from build123d import *

# Parameters (mm, degrees)
SKETCH1_R           = 32.5
BOSS_EXTRUDE1_DEPTH = 10
BOSS_EXTRUDE2_DEPTH = 5.4
SKETCH3_R           = 7
CUT_EXTRUDE1_DEPTH  = 49.473291615


with BuildPart() as part:
    # Sketch1 → Boss-Extrude1 (new body)
    with BuildSketch(Plane(origin=(0, 0, 0), x_dir=(1, 0, 0), z_dir=(0, 1, 0))):
        with Locations(Location((0, 0, 0), (0, 0, 270))):
            Circle(SKETCH1_R)
    extrude(amount=BOSS_EXTRUDE1_DEPTH)

    # Sketch2 → Boss-Extrude2 (add)
    with BuildSketch(Plane(origin=(0, 10, 0), x_dir=(1, 0, 0), z_dir=(0, 1, 0))):
        with BuildLine():
            Line((2.725, 11.891777622), (2.725, 17.25))
            Line((2.725, 17.25), (-2.725, 17.25))
            Line((-2.725, 17.25), (-2.725, 11.891777622))
            ThreePointArc((-2.725, 11.891777622), (-8.62670273, 8.62670273), (-11.891777622, 2.725))
            Line((-11.891777622, 2.725), (-17.25, 2.725))
            Line((-17.25, 2.725), (-17.25, -2.725))
            Line((-17.25, -2.725), (-11.891777622, -2.725))
            ThreePointArc((-11.891777622, -2.725), (-8.62670273, -8.62670273), (-2.725, -11.891777622))
            Line((-2.725, -11.891777622), (-2.725, -17.25))
            Line((-2.725, -17.25), (2.725, -17.25))
            Line((2.725, -17.25), (2.725, -11.891777622))
            ThreePointArc((2.725, -11.891777622), (8.62670273, -8.62670273), (11.891777622, -2.725))
            Line((11.891777622, -2.725), (17.25, -2.725))
            Line((17.25, -2.725), (17.25, 2.725))
            Line((17.25, 2.725), (11.891777622, 2.725))
            ThreePointArc((11.891777622, 2.725), (8.62670273, 8.62670273), (2.725, 11.891777622))
        make_face()
    extrude(amount=BOSS_EXTRUDE2_DEPTH)

    # Sketch3 → Cut-Extrude1 (cut, through all)
    with BuildSketch(Plane(origin=(0, 15.4, 0), x_dir=(1, 0, 0), z_dir=(0, 1, 0))):
        with Locations(Location((0, 0, 0), (0, 0, 270))):
            Circle(SKETCH3_R)
    extrude(amount=-CUT_EXTRUDE1_DEPTH, mode=Mode.SUBTRACT)


solid = part.part
Part model, mm, in its own coordinate system. A direction names the side the tool comes from. Give positions to 0.01 mm unless a question says otherwise; leave off trailing zeros. Loops run counter-clockwise (first coordinate to the right, second up) from the corner with the lowest first, then second, coordinate; pieces in that order, holes last. Notation, with made-up numbers: M 88.5,-10 L 114.5,-10 A35 cw 114.5,22 Z; hole C 68.5,3 d3. An arc over 180 degrees is marked long. Put each result on its own line as item: value. Start each with the question number.
1) Saw through at C-C (y = 12). List the corners of the cut face in (x, z) (3 decimals), then the cut area to 3 significant figures.
2) Saw through at D-D (x = 16). List the corners of the cut face in (y, z) (3 decimals).
3) Flat gauge pins, fed straight in: pin 1 (4 mm diameter, centred on x = 25, z = 7.5, fed in from -Y); pin 2 (4.5 mm diameter, centred on y = 14, z = 14.5, fed in from -X) (3 decimals); pin 3 (2.5 mm diameter, centred on x = -14.5, y = 13.5, fed in from +Z) (3 decimals); pin 4 (3 mm diameter, centred on x = 3.5, y = 12, fed in from +Z). Where does each tip first touch, or does it go through?
4) Probe probe 1 along X at (y, z) = (7.75, 0); probe 2 along Y at (x, z) = (-1, -22.5); probe 3 along Z at (x, y) = (-3, 2.25). List the from-to ranges inside material, lowest first.
5) Pull direction Z, two halves, no side cores. Call faces 4 (the flat face through (-15, 13, 2.725)), 5 (the cylindrical face through (-6.834, 7.808, -1.517)), 6 (the flat face through (-15, 13, -2.725)), 7 (the flat face through (2.725, 13, 15)): +Z half, -Z half, draft (parallel to the pull), parting line (faces both ways), or undercut.
6) 3-axis set-ups, long thin cutter, end or side, ignore diameter. For faces 1 (the cylindrical face through (-8.694, 12.662, 8.559)), 2 (the flat face through (0, 13, 17.25)), 3 (the flat face through (17.25, 13, 0)): which of +Z, -Z, +X, -X, +Y, -Y reach the whole face in a straight line?
7) Saw through at A-A (z = 0). List the corners of the cut face in (x, y).
8) Saw through at B-B (x = 0). List the corners of the cut face in (y, z), then the cut area to 3 significant figures.
Numbers:
1. outline: M -17.25,-2.725 L -11.892,-2.725 A12.2 ccw -2.725,-11.892 L -2.725,-17.25 L 2.725,-17.25 L 2.725,-11.892 A12.2 ccw 11.892,-2.725 L 17.25,-2.725 L 17.25,2.725 L 11.892,2.725 A12.2 ccw 2.725,11.892 L 2.725,17.25 L -2.725,17.25 L -2.725,11.892 A12.2 ccw -11.892,2.725 L -17.25,2.725 Z; hole C 0,0 d14
1. area: 426 mm^2
2. outline: M 0,-28.289 L 10,-28.289 L 10,-2.725 L 15.4,-2.725 L 15.4,2.725 L 10,2.725 L 10,28.289 L 0,28.289 Z
3. pin 1: y = 0
3. pin 2: x = -2.725
3. pin 3: z = 2.725
3. pin 4: z = 17.25
4. probe 1: -32.5 to -7, 7 to 32.5
4. probe 2: 0 to 10
4. probe 3: -32.36 to -6.32, 6.32 to 32.36
5. face 4: +Z half
5. face 5: undercut
5. face 6: -Z half
5. face 7: draft
6. face 1: +Z, -X, +Y
6. face 2: +Z, +X, -X, +Y
6. face 3: +Z, -Z, +X, +Y
7. outline: M -32.5,0 L -7,0 L -7,15.4 L -17.25,15.4 L -17.25,10 L -32.5,10 Z; M 7,0 L 32.5,0 L 32.5,10 L 17.25,10 L 17.25,15.4 L 7,15.4 Z
8. outline: M 0,-32.5 L 10,-32.5 L 10,-17.25 L 15.4,-17.25 L 15.4,-7 L 0,-7 Z; M 0,7 L 15.4,7 L 15.4,17.25 L 10,17.25 L 10,32.5 L 0,32.5 Z
8. area: 621 mm^2
